```python
from build123d import *

# Parameters (mm, degrees)
SKETCH1_R           = 8.1
BOSS_EXTRUDE1_DEPTH = 3


with BuildPart() as part:
    # Sketch1 → Boss-Extrude1 (new body)
    with BuildSketch(Plane(origin=(0, 0, 0), x_dir=(1, 0, 0), z_dir=(0, 1, 0))):
        Polygon((-111, 30), (-116, 30), (-116, 10), (-111, 10), (-111, -10), (-116, -10), (-116, -30), (-111, -30), (-111, -50), (-66.6, -50), (-66.6, -54), (-41, -54), (-41, -22), (-61, -22), (-61, -5), (-41, -5), (41, -5), (61, -5), (61, -22), (41, -22), (41, -54), (66.6, -54), (66.6, -50), (111, -50), (111, -30), (116, -30), (116, -10), (111, -10), (111, 10), (116, 10), (116, 30), (111, 30), (111, 50), (-111, 50), align=None)
        with Locations(Location((12.8, 15, 0), (0, 0, 270))):
            Circle(SKETCH1_R, mode=Mode.SUBTRACT)
        with Locations(Location((-12.8, 15, 0), (0, 0, 270))):
            Circle(SKETCH1_R, mode=Mode.SUBTRACT)
        with BuildLine():
            Line((-2.85, 2.4), (2.85, 2.4))
            ThreePointArc((2.85, 2.4), (7.35, 6.9), (2.85, 11.4))
            Line((2.85, 11.4), (-2.85, 11.4))
            ThreePointArc((-2.85, 11.4), (-7.35, 6.9), (-2.85, 2.4))
        make_face(mode=Mode.SUBTRACT)
    extrude(amount=BOSS_EXTRUDE1_DEPTH)


solid = part.part
```
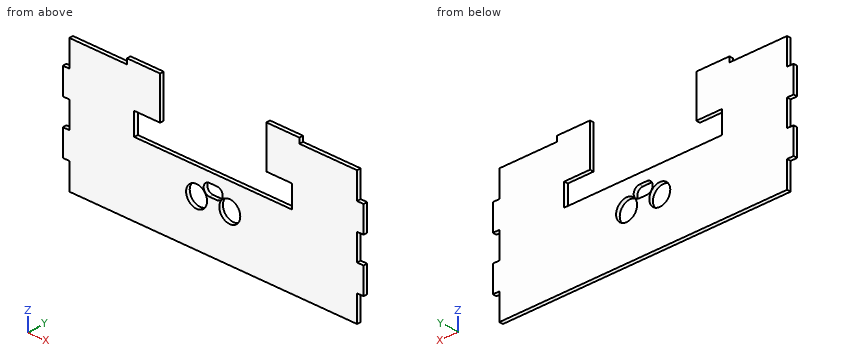
Here's how the part is built. I have some questions about the finished solid (model axes, mm). Coordinates: 2 decimals unless noted, no trailing zeros. Write each loop counter-clockwise with the first axis right and the second up, starting at its lowest first coordinate (ties: lowest second). Pieces come first, ordered by that corner, then holes. Notation, with made-up numbers: (49, 62) -> (57, 62) arc R20 ccw to (57, 88) -> close; hole circle Ø5 at (-34.5, 54). An arc over 180 degrees is marked (long way). Use a Markdown table: item, result. Add a question column.
(1) If we section it at B-B, the plane x = -47.5: Write out the boundary of the cut face in (y, z).
(2) Please list where these lines run through material, in increasing order: line 1 (X direction, y = 0.7, z = -15); line 2 (Z direction, x = -54.5, y = 1.35); line 3 (X direction, y = 2.5, z = 19.5).
(3) I'm going to push flat-ended pins straight in: P1, Ø0.9, axis at x = 96, y = 2, coming from the +Z side; P2, Ø1.5, axis at x = -114.5, y = 1.5, coming from the +Z side; P3, Ø0.9, axis at x = 113, y = 1, coming from the -Z side. Where does each tip first touch, or does it pass through?
(4) If we section it at D-D, the plane y = 2.15: State how many separate pieces and enclosed holes the cut face has, and give its area (3 significant figures).
(5) If we section it at C-C, the plane z = 44: Write out the boundary of the cut face in (x, y).
(6) If we section it at A-A, the plane z = -15: Write out the boundary of the cut face in (x, y).
Outcome:
| question | item | result |
|---|---|---|
| 1 | outline | (0, -50) -> (3, -50) -> (3, 5) -> (0, 5) -> close; (0, 22) -> (3, 22) -> (3, 54) -> (0, 54) -> close |
| 2 | line 1 | x = -116 to -20.9, -4.7 to 4.7, 20.9 to 116 |
| 2 | line 2 | z = -50 to 5, 22 to 54 |
| 2 | line 3 | x = -116 to -61, 61 to 116 |
| 3 | P1 | stops at z = 50 |
| 3 | P2 | stops at z = 30 |
| 3 | P3 | stops at z = -30 |
| 4 | separate pieces | 1 |
| 4 | enclosed holes | 3 |
| 4 | area | 17,900 mm^2 |
| 5 | outline | (-111, 0) -> (-41, 0) -> (-41, 3) -> (-111, 3) -> close; (41, 0) -> (111, 0) -> (111, 3) -> (41, 3) -> close |
| 6 | outline | (-116, 0) -> (-20.9, 0) -> (-20.9, 3) -> (-116, 3) -> close; (-4.7, 0) -> (4.7, 0) -> (4.7, 3) -> (-4.7, 3) -> close; (20.9, 0) -> (116, 0) -> (116, 3) -> (20.9, 3) -> close |
